from build123d import *

# Parameters (mm, degrees)
SKETCH1_W                    = 10
SKETCH1_H                    = 84
BASE_FLANGE1_DEPTH           = 1.75
EDGE_FLANGE1_STRIP_W         = 7.8
EDGE_FLANGE1_STRIP_H         = 1.75
EDGE_FLANGE1_STRIP_CUT_DEPTH = 84
EDGE_FLANGE1_DEPTH           = 84
SSD_MOUNTING_HOLES_D         = 2.4
SPINE_MOUNTING_HOLES_D       = 3.4
FILLET1_R                    = 3


# Sheet-metal steps are written as plain solids
with BuildPart() as part:
    # Sketch1 → Base-Flange1 (new body)
    with BuildSketch(Plane.XY):
        with Locations((5, 42)):
            Rectangle(SKETCH1_W, SKETCH1_H)
    extrude(amount=-BASE_FLANGE1_DEPTH)

    # Edge-Flange1 strip (across the edge) → Edge-Flange1 strip cut (cut)
    with BuildSketch(Plane.XZ.offset(-84)):
        with Locations((-1.75, -0.875)):
            Rectangle(EDGE_FLANGE1_STRIP_W, EDGE_FLANGE1_STRIP_H)
    extrude(amount=EDGE_FLANGE1_STRIP_CUT_DEPTH, mode=Mode.SUBTRACT)

    # Edge-Flange1 section (across the edge) → Edge-Flange1 (add)
    with BuildSketch(Plane.XZ.offset(-84)):
        with BuildLine():
            Line((0, 0.4), (0, 8.25))
            Line((0, 8.25), (1.75, 8.25))
            Line((1.75, 8.25), (1.75, 0.4))
            ThreePointArc((1.75, 0.4), (1.867157288, 0.117157288), (2.15, 0))
            Line((2.15, 0), (2.15, -1.75))
            ThreePointArc((2.15, -1.75), (0.62972042, -1.12027958), (0, 0.4))
        make_face()
    extrude(amount=EDGE_FLANGE1_DEPTH)

    # ssd-mounting-holes (through all)
    with Locations(Plane(origin=(6, 80.3, -1.75), x_dir=(-1, 0, 0), z_dir=(0, 0, -1))):
        with Locations((0, 0), (0, -76.6)):
            Hole(SSD_MOUNTING_HOLES_D / 2)

    # spine-mounting-holes (through all)
    with Locations(Plane(origin=(1.75, 0, 0), x_dir=(0, 0, -1), z_dir=(1, 0, 0))):
        with Locations((-4.325, 80.3), (-4.325, 3.7)):
            Hole(SPINE_MOUNTING_HOLES_D / 2)

    # Fillet1
    fillet1_edges = [part.edges().sort_by_distance(p)[0] for p in [
        (0.875, 84, 8.25),
        (0.875, 0, 8.25),
        (10, 84, -0.875),
        (10, 0, -0.875),
    ]]
    fillet(fillet1_edges, radius=FILLET1_R)


solid = part.part
Can you work these out from the model? Positions are in its coordinate system, mm. A direction names the side the tool comes from. Give positions to 0.01 mm unless a question says otherwise; leave off trailing zeros. Order: outer loops, then holes, each group sorted by start corner. A loop starts at its lowest first (then second) coordinate and runs counter-clockwise, first axis right, second up. Notation, with made-up numbers: M 47.5,76.25 L 66.5,76.25 A16 cw 66.5,102.25 Z; hole C -16,83 d6. An arc over 180 degrees is marked long. Use one line per item in the form item = value. Start each with the question number.
Item 1: If I drill on line 1 along Y through (x, z) = (6, -1.25); line 2 along Z through (x, y) = (3.75, 78); line 3 along X through (y, z) = (67, 1), over which ranges is the centre line in solid material (lowest first)?
Item 2: If we section it at A-A (x = 6): Write out the boundary of the cut face in (y, z), then the cut area to 3 significant figures.
Item 3: If we section it at D-D (y = 52.5): Write out the boundary of the cut face in (x, z), then the cut area to 3 significant figures.
Item 4: Will these pins go through, and if not, where does the flat tip stop? pin 1 Ø1.5 at (y, z) = (32, 4.5) entering from +X; pin 2 Ø3 at (x, y) = (6, 3.7) entering from +Z; pin 3 Ø1.5 at (x, z) = (7.5, 1) entering from +Y.
Item 5: For faces 1 (the cylindrical face through (5.74, 2.53, -0.86)), 2 (the flat face through (6, 43, 0)), which set-ups out of +Z, -Z, +X, -X, +Y, -Y let a thin tool reach every point of the face, with its end or its side?
Item 6: If we section it at C-C (z = 3.75): Write out the boundary of the cut face in (x, y), then the cut area to 3 significant figures.
Item 7: We'd pull the mould along Z, two halves only. Please class faces 3 (the cylindrical face through (0.65, 42.59, -1.14)), 4 (the flat face through (0, 43, 4)), 5 (the cylindrical face through (0.863, 81.986, 4.104)), 6 (the cylindrical face through (0.89, 83.14, 7.35)): +Z half, -Z half, draft (parallel to the pull), parting line (faces both ways), or undercut.
Item 8: If we section it at B-B (y = 3.7): Write out the boundary of the cut face in (x, z) (3 decimals).
Outcome:
q1.line_1 = 0 to 2.5, 4.9 to 79.1, 81.5 to 84
q1.line_2 = -1.75 to 0
q1.line_3 = 0 to 1.75
q2.outline = M 0,-1.75 L 2.5,-1.75 L 2.5,0 L 0,0 Z; M 4.9,-1.75 L 79.1,-1.75 L 79.1,0 L 4.9,0 Z; M 81.5,-1.75 L 84,-1.75 L 84,0 L 81.5,0 Z
q2.area = 139 mm2
q3.outline = M 0,0.4 A2.15 ccw 2.15,-1.75 L 10,-1.75 L 10,0 L 2.15,0 A0.4 cw 1.75,0.4 L 1.75,8.25 L 0,8.25 Z
q3.area = 31.0 mm2
q4.pin_1 = 1.75
q4.pin_2 = 0
q4.pin_3 = through
q5.face_1 = +Z, -Z
q5.face_2 = +Z, +X, +Y, -Y
q6.outline = M 0,0 L 1.75,0 L 1.75,2.1 L 0,2.1 Z; M 0,5.3 L 1.75,5.3 L 1.75,78.7 L 0,78.7 Z; M 0,81.9 L 1.75,81.9 L 1.75,84 L 0,84 Z
q6.area = 136 mm2
q7.face_3 = -Z half
q7.face_4 = draft
q7.face_5 = undercut
q7.face_6 = +Z half
q8.outline = M 0,0.4 A2.15 ccw 2.15,-1.75 L 4.8,-1.75 L 4.8,0 L 2.15,0 A0.4 cw 1.75,0.4 L 1.75,2.625 L 0,2.625 Z; M 0,6.025 L 1.75,6.025 L 1.75,8.25 L 0,8.25 Z; M 7.2,-1.75 L 10,-1.75 L 10,0 L 7.2,0 Z
